```python
from build123d import *

# Parameters (mm, degrees)
SZKIC1_R                    = 20
DODANIE_WYCI_GNI_CIE1_DEPTH = 58
SZKIC3_R                    = 31
DODANIE_WYCI_GNI_CIE2_DEPTH = 12
SZKIC4_W                    = 39.24283374
SZKIC4_H                    = 7
WYTNIJ_WYCI_GNI_CIE1_DEPTH  = 12
SZKIC5_R                    = 12.35
WYTNIJ_WYCI_GNI_CIE2_DEPTH  = 70
SZKIC6_R                    = 3
WYTNIJ_WYCI_GNI_CIE3_DEPTH  = 12
SFAZOWANIE1_SIZE            = 0.5


with BuildPart() as part:
    # Szkic1 → Dodanie-wyciągnięcie1 (new body)
    with BuildSketch(Plane.XY):
        Circle(SZKIC1_R)
    extrude(amount=DODANIE_WYCI_GNI_CIE1_DEPTH)

    # Szkic3 → Dodanie-wyciągnięcie2 (add)
    with BuildSketch(Plane(origin=(0, 0, 0), x_dir=(-1, 0, 0), z_dir=(0, 0, -1))):
        Circle(SZKIC3_R)
    extrude(amount=DODANIE_WYCI_GNI_CIE2_DEPTH)

    # Szkic4 → Wytnij-wyciągnięcie1 (cut)
    with BuildSketch(Plane(origin=(0, 0, -12), x_dir=(-1, 0, 0), z_dir=(0, 0, -1))):
        with Locations((0, -27.5)):
            Rectangle(SZKIC4_W, SZKIC4_H)
    extrude(amount=-WYTNIJ_WYCI_GNI_CIE1_DEPTH, mode=Mode.SUBTRACT)

    # Szkic5 → Wytnij-wyciągnięcie2 (cut)
    with BuildSketch(Plane(origin=(0, 0, -12), x_dir=(-1, 0, 0), z_dir=(0, 0, -1))):
        Circle(SZKIC5_R)
    extrude(amount=-WYTNIJ_WYCI_GNI_CIE2_DEPTH, mode=Mode.SUBTRACT)

    # Szkic6 → Wytnij-wyciągnięcie3 (cut)
    with BuildSketch(Plane(origin=(0, 0, -12), x_dir=(-1, 0, 0), z_dir=(0, 0, -1))):
        with Locations((-17.5, 17.5)):
            Circle(SZKIC6_R)
        with Locations((-25, 0)):
            Circle(SZKIC6_R)
        with Locations((-17.5, -17.5)):
            Circle(SZKIC6_R)
        with Locations((17.5, -17.5)):
            Circle(SZKIC6_R)
        with Locations((25, 0)):
            Circle(SZKIC6_R)
        with Locations((17.5, 17.5)):
            Circle(SZKIC6_R)
    extrude(amount=-WYTNIJ_WYCI_GNI_CIE3_DEPTH, mode=Mode.SUBTRACT)

    # Sfazowanie1
    sfazowanie1_edges = [part.edges().sort_by_distance(p)[0] for p in [
        (-14.5, 17.5, 0),
        (-14.5, 17.5, -12),
        (-22, 0, 0),
        (-22, 0, -12),
        (-14.5, -17.5, 0),
        (-14.5, -17.5, -12),
        (28, 0, 0),
        (28, 0, -12),
        (20.5, -17.5, 0),
        (20.5, -17.5, -12),
        (20.5, 17.5, 0),
        (20.5, 17.5, -12),
    ]]
    chamfer(sfazowanie1_edges, length=SFAZOWANIE1_SIZE)


solid = part.part
```
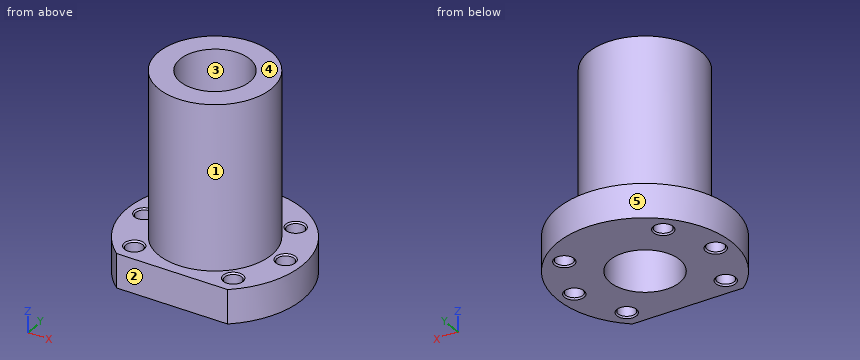
Work out the finished part from the listing and answer in its coordinate system (mm). Face numbers are marked on the shaded views. A direction names the side the tool comes from. Round coordinates to 2 decimals unless told otherwise and drop trailing zeros. Write each loop counter-clockwise with the first axis right and the second up, starting at its lowest first coordinate (ties: lowest second). Pieces come first, ordered by that corner, then holes. Notation, with made-up numbers: (63, 76.5) -> (77, 76.5) arc R27 cw to (77, 96.5) -> close; hole circle Ø2 at (38, 43). An arc over 180 degrees is marked (long way). Write each question's results on one line, items separated by ' | '.
Q1. Section B-B, the plane x = 0 is taken. Write down the section's boundary in (y, z).
Data:
outline: (-24, -12) -> (-12.35, -12) -> (-12.35, 58) -> (-20, 58) -> (-20, 0) -> (-24, 0) -> close; (12.35, -12) -> (31, -12) -> (31, 0) -> (20, 0) -> (20, 58) -> (12.35, 58) -> close
Q2. Section A-A, the plane y = 0 is taken. Write down the section's boundary in (x, z).
Data:
outline: (-31, -12) -> (-28.5, -12) -> (-28, -11.5) -> (-28, -0.5) -> (-28.5, 0) -> (-31, 0) -> close; (-22, -11.5) -> (-21.5, -12) -> (-12.35, -12) -> (-12.35, 58) -> (-20, 58) -> (-20, 0) -> (-21.5, 0) -> (-22, -0.5) -> close; (12.35, -12) -> (21.5, -12) -> (22, -11.5) -> (22, -0.5) -> (21.5, 0) -> (20, 0) -> (20, 58) -> (12.35, 58) -> close; (28, -11.5) -> (28.5, -12) -> (31, -12) -> (31, 0) -> (28.5, 0) -> (28, -0.5) -> close
Q3. Determine the mould class of the marked faces 3, 4 and 5 for opening direction Y: released by +Y, released by -Y, zero draft, split by the parting line, or undercut.
Data:
face 3: undercut | face 4: zero draft | face 5: split by the parting line
Q4. Straight lines are drawn through the part: line 1 along X through (y, z) = (-17, -6); line 2 along Y through (x, z) = (0, 18.5); line 3 along Y through (x, z) = (17.5, -7.5). For each, find the intervals that lie inside material, in ascending order. Write a range as [from, to].
Data:
line 1: [-25.92, -20.46], [-14.54, 14.54], [20.46, 25.92] | line 2: [-20, -12.35], [12.35, 20] | line 3: [-24, -20.5], [-14.5, 14.5], [20.5, 25.59]
Q5. Which of the six approach directions +Z, -Z, +X, -X, +Y, -Y give full straight-line access (tool end or side, diameter ignored) to the marked faces 1 and 2?
Data:
face 1: +Z | face 2: +Z, -Z, +X, -X, -Y
Q6. Section D-D, the plane y = -7.5 is taken. Write down the section's boundary in (x, z), then the cut area to 3 significant figures.
Data:
outline: (-30.08, -12) -> (-9.81, -12) -> (-9.81, 58) -> (-18.54, 58) -> (-18.54, 0) -> (-30.08, 0) -> close; (9.81, -12) -> (30.08, -12) -> (30.08, 0) -> (18.54, 0) -> (18.54, 58) -> (9.81, 58) -> close | area: 1,500 mm^2
Q7. Section C-C, the plane x = 17.5 is taken. Write down the section's boundary in (y, z), then the cut area to 3 significant figures.
Data:
outline: (-24, -12) -> (-21, -12) -> (-20.5, -11.5) -> (-20.5, -0.5) -> (-21, 0) -> (-24, 0) -> close; (-14.5, -11.5) -> (-14, -12) -> (14, -12) -> (14.5, -11.5) -> (14.5, -0.5) -> (14, 0) -> (9.68, 0) -> (9.68, 58) -> (-9.68, 58) -> (-9.68, 0) -> (-14, 0) -> (-14.5, -0.5) -> close; (20.5, -11.5) -> (21, -12) -> (25.59, -12) -> (25.59, 0) -> (21, 0) -> (20.5, -0.5) -> close | area: 1,570 mm^2
Q8. Flat-ended cylindrical pins translate along their axes: P1, Ø5, axis at x = -17.5, y = -17.5, coming from the -Z side; P2, Ø16.5, axis at x = 6, y = -4, coming from the +Z side; P3, Ø8, axis at x = 8.5, z = 40, coming from the -Y side; P4, Ø2, axis at x = 0, z = 41.5, coming from the +Y side. Find the tip coordinate at first contact, or state that the pin passes through.
Data:
P1: through | P2: z = 58 | P3: y = -19.49 | P4: y = 20
